Autodesk Inventor part; units mm, degrees
ref_plane "Work Plane1" through (0, 0, 61.9125) normal (0, 0, 1) x (1, 0, 0)
ref_plane "Work Plane2" through (0, 0, 7.9375) normal (0, 0, -1) x (-1, 0, 0)
ref_plane "Work Plane3" through (0, 0, 44.2214) normal (0, 0, 1) x (1, 0, 0)
sketch "Sketch1" plane through (0, 0, 0) normal (0, 0, 1) x (1, 0, 0)
  circle A0 centre (0, 0) radius 4.7625
  line L0 (-1.5875, 6.35) -> (1.5875, 6.35)
  line L1 (1.5875, 6.35) -> (1.5875, 3.175)
  line L2 (1.5875, 3.175) -> (-1.5875, 3.175)
  line L3 (-1.5875, 3.175) -> (-1.5875, 6.35)
  dimension "d0" = 9.525
  dimension "d16" = 3.175
  dimension "d17" = 3.175
  dimension "d18" = 1.5875
  dimension "d19" = 6.35
extrude "Extrusion1" add sketch "Sketch1" along normal blind 69.85 contours A0 L3 L2 L1 | L1 L2 L3 A0
ref_plane "Work Plane1" through (0, 0, 61.9125) normal (0, 0, 1) x (1, 0, 0)
sketch "Sketch2" plane through (0, 0, 61.9125) normal (0, 0, 1) x (1, 0, 0)
  circle A0 centre (0, 0) radius 3.81
  circle A1 centre (0, 0) radius 4.7625
  dimension "d4" = 7.62
extrude "Extrusion2" cut sketch "Sketch2" against normal blind 1.143
ref_plane "Work Plane2" through (0, 0, 7.9375) normal (0, 0, -1) x (-1, 0, 0)
sketch "Sketch3" plane through (0, 0, 7.9375) normal (0, 0, -1) x (-1, 0, 0)
  circle A0 centre (0, 0) radius 3.81
  circle A1 centre (0, 0) radius 4.7625
extrude "Extrusion3" cut sketch "Sketch3" against normal blind 1.143
ref_plane "Work Plane3" through (0, 0, 44.2214) normal (0, 0, 1) x (1, 0, 0)
sketch "Sketch4" plane through (0, 0, 44.2214) normal (0, 0, 1) x (1, 0, 0)
  circle A0 centre (0, 0) radius 3.81
  circle A1 centre (0, 0) radius 4.7625
extrude "Extrusion4" cut sketch "Sketch4" along normal blind 1.143
ref_plane "Work Plane4" through (0, 0, 68.1736) normal (0, 0, 1) x (1, 0, 0)
extrude "Extrusion6" cut sketch "Sketch1" along normal through all contours L1 L2 L3 A0 | A0 L3 L0 L1 picked at (-0.1794, 3.694)
equation "\"d17\" = d16"
properties part number "lower box upper shaft"
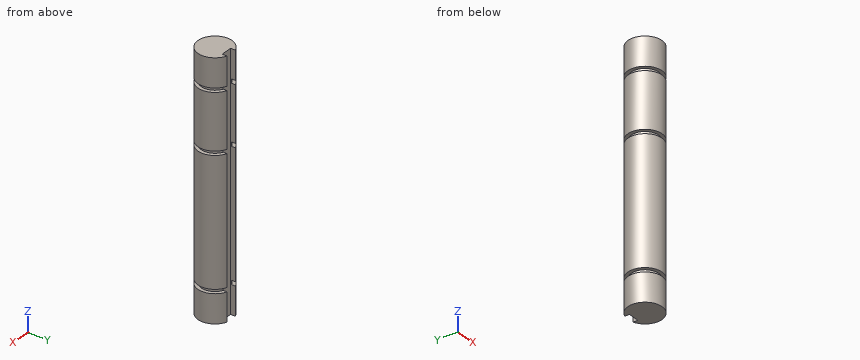
The listing builds one solid part. Answer for the finished solid, in the listing's coordinates (mm). Give positions to 0.01 mm unless a question says otherwise; leave off trailing zeros. Order: outer loops, then holes, each group sorted by start corner. A loop starts at its lowest first (then second) coordinate and runs counter-clockwise, first axis right, second up. Notation, with made-up numbers: (79, -35.5) - (105, -35.5) arc R28 ccw to (105, 1.5) - close; hole circle Ø9 at (33.25, 18.5). An arc over 180 degrees is marked (long way). One line per item, written item: value. Start each with the question number.
1) A cutting plane is placed at C-C on z = 12.5. Give the vertices of the cut face in (x, y) (1 decimal).
2) Given pin 1 Ø1.5 at (x, z) = (2.5, 30) entering from -Y; pin 2 Ø1 at (x, z) = (-0.5, 39.5) entering from +Y (3 decimals), each flat-ended and moving along its own axis, determine where each tip first touches the part or whether it passes through.
3) A cutting plane is placed at B-B on y = 1. Give the vertices of the cut face in (x, z).
4) Find the intervals of material crossed by L1, parallel to Z at x = 3.25, y = -2.25; L2, parallel to Y at x = 0, z = 44 (1 decimal); L3, parallel to Y at x = -0.75, z = 28.5 (3 decimals), in increasing order.
5) A cutting plane is placed at D-D on x = 3. Give the vertices of the cut face in (y, z).
Answer sheet:
1. outline: (-1.6, 3.2) - (-1.6, 4.5) arc R4.8 ccw (long way) to (1.6, 4.5) - (1.6, 3.2) - close
2. pin 1: stops at y = -4.43
2. pin 2: stops at y = 3.175
3. outline: (-4.66, 0) - (4.66, 0) - (4.66, 7.94) - (3.68, 7.94) - (3.68, 9.08) - (4.66, 9.08) - (4.66, 44.22) - (3.68, 44.22) - (3.68, 45.36) - (4.66, 45.36) - (4.66, 60.77) - (3.68, 60.77) - (3.68, 61.91) - (4.66, 61.91) - (4.66, 69.85) - (-4.66, 69.85) - (-4.66, 61.91) - (-3.68, 61.91) - (-3.68, 60.77) - (-4.66, 60.77) - (-4.66, 45.36) - (-3.68, 45.36) - (-3.68, 44.22) - (-4.66, 44.22) - (-4.66, 9.08) - (-3.68, 9.08) - (-3.68, 7.94) - (-4.66, 7.94) - close
4. L1: z = 0 to 7.94, 9.08 to 44.22, 45.36 to 60.77, 61.91 to 69.85
4. L2: y = -4.8 to 3.2
4. L3: y = -4.703 to 3.175
5. outline: (-3.7, 0) - (3.7, 0) - (3.7, 7.94) - (2.35, 7.94) - (2.35, 9.08) - (3.7, 9.08) - (3.7, 44.22) - (2.35, 44.22) - (2.35, 45.36) - (3.7, 45.36) - (3.7, 60.77) - (2.35, 60.77) - (2.35, 61.91) - (3.7, 61.91) - (3.7, 69.85) - (-3.7, 69.85) - (-3.7, 61.91) - (-2.35, 61.91) - (-2.35, 60.77) - (-3.7, 60.77) - (-3.7, 45.36) - (-2.35, 45.36) - (-2.35, 44.22) - (-3.7, 44.22) - (-3.7, 9.08) - (-2.35, 9.08) - (-2.35, 7.94) - (-3.7, 7.94) - close
